Here's how the part is built. I have some questions about the finished solid (model axes, mm). Face numbers are marked on the shaded views. A direction names the side the tool comes from. Coordinates: 2 decimals unless noted, no trailing zeros. Write each loop counter-clockwise with the first axis right and the second up, starting at its lowest first coordinate (ties: lowest second). Pieces come first, ordered by that corner, then holes.
Item 1: If I drill on line 1 (Y direction, x = -0.75, z = -2); line 2 (Z direction, x = -1.25, y = -2); line 3 (X direction, y = 1.5, z = 1), over which ranges is the centre line in solid material (lowest first)?
Item 2: I'm going to push flat-ended pins straight in: pin 1 Ø1.9 at (y, z) = (14.5, -2) entering from +X; pin 2 Ø0.5 at (x, y) = (1.5, 14.5) entering from +Z; pin 3 Ø0.5 at (x, y) = (-1.5, 13.5) entering from -Z. Where does each tip first touch, or does it pass through?
Item 3: If we section it at B-B (y = 7): Please give me the cut outline in (x, z).
Item 4: If we section it at A-A (x = 0): Please give me the cut outline in (y, z).
Item 5: For the marked faces 1 and 2, which set-ups out of +Z, -Z, +X, -X, +Y, -Y let a thin tool reach every point of the face, with its end or its side?
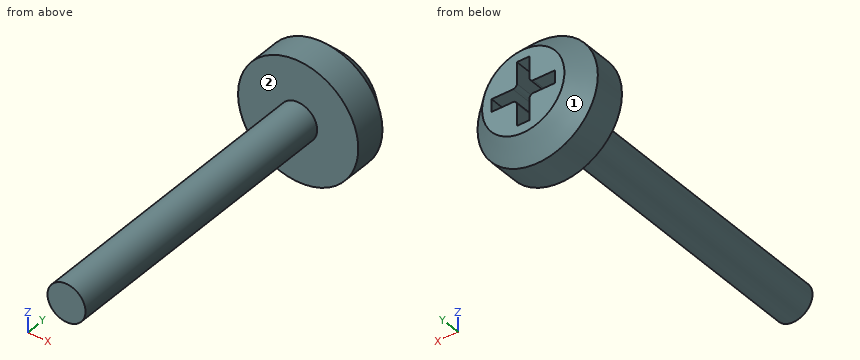
from build123d import *

# Parameters (mm, degrees)
F0_R      = 1.5
F1_DEPTH  = 12
F2_R      = 4.75
F2_R_2    = 1.5
F3_DEPTH  = 2.5
F5_R      = 3.25
F3_FACE_R = 4.75
F7_W      = 1
F7_H      = 2
F7_H_2    = 1
F7_W_2    = 2
F8_DEPTH  = 3.9
F9_R      = 0.3


with BuildPart() as f1:
    # F0 (on Front) → F1 (new body, symmetric)
    with BuildSketch(Plane.XZ):
        Circle(F0_R)
    extrude(amount=F1_DEPTH, both=True)

    # F2 (on face) → F3 (join)
    with BuildSketch(Plane(origin=(0, 12, 0), x_dir=(-1, 0, 0), z_dir=(0, 1, 0))):
        Circle(F2_R)
        Circle(F2_R_2, mode=Mode.SUBTRACT)
        Circle(F2_R_2)
    extrude(amount=F3_DEPTH)

    # F5 (on offset) → F6 section 0
    with BuildSketch(Plane.XZ.offset(-16)):
        Circle(F5_R)
    # F3_face (on face) → F6 section 1
    with BuildSketch(Plane(origin=(0, 14.5, 0), x_dir=(-1, 0, 0), z_dir=(0, 1, 0))):
        Circle(F3_FACE_R)
    loft()

    # F7 (on face) → F8 (cut)
    with BuildSketch(Plane(origin=(0, 16, 0), x_dir=(-1, 0, 0), z_dir=(0, 1, 0))):
        with Locations((0, -1.5)):
            Rectangle(F7_W, F7_H)
        Rectangle(F7_W, F7_H_2)
        with Locations((-1.5, 0)):
            Rectangle(F7_W_2, F7_H_2)
        with Locations((0, 1.5)):
            Rectangle(F7_W, F7_H)
        with Locations((1.5, 0)):
            Rectangle(F7_W_2, F7_H_2)
    extrude(amount=-F8_DEPTH, mode=Mode.SUBTRACT)

    # F9
    f9_edges = [f1.edges().sort_by_distance(p)[0] for p in [
        (-0.5, 14.05, 0.5),
        (0.5, 14.05, 0.5),
        (0.5, 14.05, -0.5),
        (-0.5, 14.05, -0.5),
    ]]
    fillet(f9_edges, radius=F9_R)


solid = f1.part
Answer list:
1. line 1: y = 12 to 16
1. line 2: z = -0.83 to 0.83
1. line 3: x = -1.12 to 1.12
2. pin 1: stops at x = 4.63
2. pin 2: stops at z = 4.58
2. pin 3: stops at z = -4.58
3. outline: circle Ø3 at (0, 0)
4. outline: (-12, -1.5) - (12, -1.5) - (12, -4.75) - (14.5, -4.75) - (16, -3.25) - (16, -2.5) - (12.1, -2.5) - (12.1, 2.5) - (16, 2.5) - (16, 3.25) - (14.5, 4.75) - (12, 4.75) - (12, 1.5) - (-12, 1.5) - close
5. face 1: +Y
5. face 2: -Y
